Design review of the part built by this model. Coordinates are the model's own, in mm. Face numbers are marked on the shaded views. A direction names the side the tool comes from. Coordinates: 2 decimals unless noted, no trailing zeros. Order: outer loops, then holes, each group sorted by start corner. A loop starts at its lowest first (then second) coordinate and runs counter-clockwise, first axis right, second up.
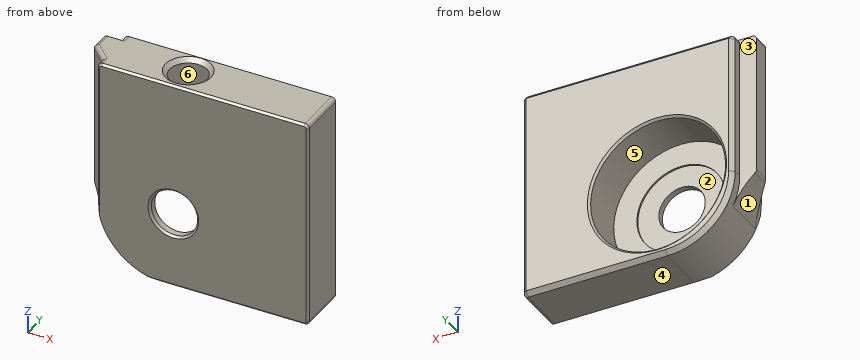
from build123d import *

# Parameters (mm, degrees)
SKETCH1_W           = 25
SKETCH1_H           = 25
BOSS_EXTRUDE1_DEPTH = 6.5
SKETCH2_R           = 8
CUT_EXTRUDE1_DEPTH  = 5.5
FILLET1_R           = 8
SKETCH4_R           = 2.2
CUT_EXTRUDE2_DEPTH  = 7.5
BOSS_EXTRUDE2_DEPTH = 17
FILLET2_R           = 10
SKETCH6_R           = 2.75
CUT_EXTRUDE3_DEPTH  = 20.918584287
BOSS_EXTRUDE3_START = 0.2
SKETCH7_R           = 8
SKETCH7_R_2         = 5.25
BOSS_EXTRUDE3_DEPTH = 0.2
FILLET3_R           = 0.5
CHAMFER1_SIZE       = 0.5
CHAMFER7_SIZE       = 0.25


# Some blends are built 0.0001 mm under size
with BuildPart() as part:
    # Sketch1 → Boss-Extrude1 (new body)
    with BuildSketch(Plane(origin=(0, 0, 0), x_dir=(1, 0, 0), z_dir=(0, 1, 0))):
        Rectangle(SKETCH1_W, SKETCH1_H)
    extrude(amount=BOSS_EXTRUDE1_DEPTH)

    # Sketch2 → Cut-Extrude1 (cut)
    with BuildSketch(Plane(origin=(0, 6.5, 0), x_dir=(1, 0, 0), z_dir=(0, 1, 0))):
        with Locations(Location((-3.5, 3.5, 0), (0, 0, 270))):
            Circle(SKETCH2_R)
    extrude(amount=-CUT_EXTRUDE1_DEPTH, mode=Mode.SUBTRACT)

    # Fillet1
    fillet1_edges = [part.edges().sort_by_distance(p)[0] for p in [
        (-12.5, 3.25, -12.5),
    ]]
    fillet(fillet1_edges, radius=FILLET1_R)

    # Sketch4 → Cut-Extrude2 (cut)
    with BuildSketch(Plane.XY.offset(12.5)):
        with Locations((-3.5, 3.25)):
            Circle(SKETCH4_R)
    extrude(amount=-CUT_EXTRUDE2_DEPTH, mode=Mode.SUBTRACT)

    # Sketch5 → Boss-Extrude2 (add)
    with BuildSketch(Plane.XY.offset(12.5)):
        Polygon((-12.5, 1), (-14.5, 3), (-14.5, 5), (-12.5, 5), align=None)
    extrude(amount=-BOSS_EXTRUDE2_DEPTH)

    # Fillet2
    # the kernel refuses this fillet: 10 mm, written as the material it adds along each edge
    with BuildSketch(Plane(origin=(-12.5, 5, -4.5), x_dir=(0.22360679774997813, 0, -0.9746794344808967), z_dir=(0, -1, 0))) as fillet2_piece_1_section:
        with BuildLine():
            CenterArc((5.813776741, -9.746794345), FILLET2_R, 102.920966382, 25.841932763)
            Line((-0.447213595, -1.949358869), (-0.572433402, -1.793410159))
            ThreePointArc((-0.572433402, -1.793410159), (-0.418542685, -0.929958075), (-0.194935887, 0.04472136))
            Line((-0.194935887, 0.04472136), (0.04472136, 0.194935887))
            ThreePointArc((0.04472136, 0.194935887), (1.788854382, -0.002564524), (3.532987404, 0.194935887))
            Line((3.532987404, 0.194935887), (3.577708764, 0))
        make_face()
    fillet2_piece_1 = extrude(amount=12.94427191, mode=Mode.PRIVATE)
    fillet2_piece_1 = split(fillet2_piece_1, bisect_by=Plane(origin=(-14.5, 3, -4.5), z_dir=(0.7071067811865512, 0.7071067811865438, 0)), keep=Keep.TOP, mode=Mode.PRIVATE)
    add(fillet2_piece_1)

    # Sketch6 → Cut-Extrude3 (cut, through all)
    with BuildSketch(Plane(origin=(0, 1, 0), x_dir=(1, 0, 0), z_dir=(0, 1, 0))):
        with Locations(Location((-3.5, 3.5, 0), (0, 0, 270))):
            Circle(SKETCH6_R)
    extrude(amount=-CUT_EXTRUDE3_DEPTH, mode=Mode.SUBTRACT)

    # Sketch7 → Boss-Extrude3 (add)
    with BuildSketch(Plane(origin=(0, 1, 0), x_dir=(1, 0, 0), z_dir=(0, 1, 0)).offset(BOSS_EXTRUDE3_START)):
        with Locations(Location((-3.5, 3.5, 0), (0, 0, 270))):
            Circle(SKETCH7_R)
        with Locations(Location((-3.5, 3.5, 0), (0, 0, 270))):
            Circle(SKETCH7_R_2, mode=Mode.SUBTRACT)
    extrude(amount=-BOSS_EXTRUDE3_DEPTH)

    # Fillet3
    fillet3_edges = [part.edges().sort_by_distance(p)[0] for p in [
        (-14.5, 4, -4.5),
        (-12.5, 0.5, 12.5),
        (-13.5, 2, 12.5),
        (-14.5, 4, 12.5),
        (-12.5, 5.75, 12.5),
        (12.5, 3.25, -12.5),
        (12.5, 3.25, 12.5),
    ]]
    fillet(fillet3_edges, radius=FILLET3_R)

    # Chamfer1
    chamfer1_edges = [part.edges().sort_by_distance(p)[0] for p in [
        (0, 6.5, 12.5),
        (3.75, 6.5, -12.5),
        (12.5, 6.5, 0),
        (12.353553391, 6.5, 12.353553391),
        (12.353553391, 6.5, -12.353553391),
        (-12.353553391, 6.5, 12.353553391),
        (-12.5, 6.5, 3.75),
        (-10.156854249, 6.5, -10.156854249),
        (-5.7, 3.25, 12.5),
    ]]
    chamfer(chamfer1_edges, length=CHAMFER1_SIZE - 0.0001)  # a hair under: the kernel refuses the full size

    # Chamfer7
    # the kernel refuses this chamfer: 0.25 mm, written as the material it takes off along each edge
    with BuildSketch(Plane(origin=(-3.5, 0, -3.5), x_dir=(0, 0, 1), z_dir=(-1, 0, 0))) as chamfer7_piece_1:
        Polygon((2.75 + CHAMFER7_SIZE, 0), (2.75, CHAMFER7_SIZE), (2.75, 0), align=None)
    revolve(axis=Axis((-3.5, 0, -3.5), (0, 1, 0)), mode=Mode.SUBTRACT)
    with BuildSketch(Plane(origin=(-12.5, 0, -7.714603735), x_dir=(1, 0, 0), z_dir=(0, 0, 1)), Plane(origin=(12, 0, -12.5), x_dir=(0, 0, 1), z_dir=(-1, 0, 0))) as chamfer7_piece_2:
        Polygon((CHAMFER7_SIZE, 0), (0, CHAMFER7_SIZE), (0, 0), align=None)
    extrude(amount=19.714603735, mode=Mode.SUBTRACT)
    with BuildSketch(Plane(origin=(-12, 0, 12.5), x_dir=(0, 1, 0), z_dir=(1, 0, 0))) as chamfer7_piece_3:
        Polygon((CHAMFER7_SIZE, 0), (0, -CHAMFER7_SIZE), (0, 0), align=None)
    extrude(amount=24, mode=Mode.SUBTRACT)
    with BuildSketch(Plane(origin=(12.5, 0, 12), x_dir=(-1, 0, 0), z_dir=(0, 0, -1))) as chamfer7_piece_4:
        Polygon((CHAMFER7_SIZE, 0), (0, CHAMFER7_SIZE), (0, 0), align=None)
    extrude(amount=24, mode=Mode.SUBTRACT)
    with BuildSketch(Plane(origin=(-3.5, 6.5, -3.5), x_dir=(0, 0, 1), z_dir=(-1, 0, 0))) as chamfer7_piece_5:
        Polygon((8 + CHAMFER7_SIZE, 0), (8, -CHAMFER7_SIZE), (8, 0), align=None)
    revolve(axis=Axis((-3.5, 6.5, -3.5), (0, 1, 0)), mode=Mode.SUBTRACT)
    with BuildSketch(Plane(origin=(12, 0, -12), x_dir=(0, 0, -1), z_dir=(-1, 0, 0))) as chamfer7_piece_6:
        Polygon((0.5 - CHAMFER7_SIZE, 0), (0.5, -CHAMFER7_SIZE), (0.5, 0), align=None)
    revolve(axis=Axis((12, 0, -12), (0, -1, 0)), revolution_arc=90, mode=Mode.SUBTRACT)
    with BuildSketch(Plane(origin=(12, 0, 12), x_dir=(0, 0, 1), z_dir=(-1, 0, 0))) as chamfer7_piece_7:
        Polygon((0.5, CHAMFER7_SIZE), (0.5 - CHAMFER7_SIZE, 0), (0.5, 0), align=None)
    revolve(axis=Axis((12, 0, 12), (0, 1, 0)), revolution_arc=90, mode=Mode.SUBTRACT)
    with BuildSketch(Plane(origin=(-12, 0, 12), x_dir=(0, 0, 1), z_dir=(1, 0, 0))) as chamfer7_piece_8:
        Polygon((0.5 - CHAMFER7_SIZE, 0), (0.5, -CHAMFER7_SIZE), (0.5, 0), align=None)
    revolve(axis=Axis((-12, 0, 12), (0, -1, 0)), revolution_arc=90, mode=Mode.SUBTRACT)


solid = part.part
1. Add section A-A (z = -3.5). Give the boundary of the cut face in (x, y), and give its area (3 significant figures).
2. To check wall thickness, follow line 1 (X direction, y = 0.85, z = -3.5); line 2 (Y direction, x = -3.5, z = 10); line 3 (Y direction, x = -1.75, z = 1.5). State the ranges of each line that lie inside material, in increasing order.
3. Add section C-C (z = 10.75). Give the boundary of the cut face in (x, y), and give its area (3 significant figures).
4. For the marked faces 4, 5 and 6, list the 3-axis set-ups (+Z, -Z, +X, -X, +Y, -Y) from which the entire face can be reached by the end or side of a thin tool; tool diameter is ignored.
5. Mouldability with a two-part tool opening along Z and no side actions: class the marked faces 1, 2 and 3 as pulls with the +Z half, pulls with the -Z half, needs draft (parallel to the pull), parting line crosses it, or undercut.
6. Insertion check: pin 1 (0.8 mm diameter, centred on y = 5.5, z = 3.5, fed in from -X); pin 2 (2 mm diameter, centred on x = -6, z = 2, fed in from -Y); pin 3 (3.5 mm diameter, centred on x = -3.5, z = -3.5, fed in from +Y); pin 4 (0.8 mm diameter, centred on x = -13.5, z = 5.5, fed in from +Y). Each pin has a flat end and moves straight along its axis. Give the tip position at first contact, or say it passes through.
Solution:
1. outline: (-14.5, 3) - (-12.5, 1) - (-12.5, 0.25) - (-12.25, 0) - (-6.5, 0) - (-6.25, 0.25) - (-6.25, 1) - (-8.75, 1) - (-8.75, 1.2) - (-11.5, 1.2) - (-11.5, 6.25) - (-11.75, 6.5) - (-12, 6.5) - (-12.5, 6) - (-12.5, 5) - (-14.5, 5) - close; (-0.75, 0.25) - (-0.5, 0) - (12.25, 0) - (12.5, 0.25) - (12.5, 6) - (12, 6.5) - (4.75, 6.5) - (4.5, 6.25) - (4.5, 1.2) - (1.75, 1.2) - (1.75, 1) - (-0.75, 1) - close
1. area: 75.7 mm2
2. line 1: x = -12.5 to -6.25, -0.75 to 12.5
2. line 2: y = 0 to 1.05, 5.45 to 6.5
2. line 3: y = 0 to 1.2
3. outline: (-14.5, 3) - (-12.5, 1) - (-12.5, 0.25) - (-12.25, 0) - (12.25, 0) - (12.5, 0.25) - (12.5, 6) - (12, 6.5) - (-12, 6.5) - (-12.5, 6) - (-12.5, 5) - (-14.5, 5) - close; hole circle Ø4.4 at (-3.5, 3.25)
3. area: 153 mm2
4. face 4: -Z, +X, -X, +Y, -Y
4. face 5: +Y
4. face 6: +Z
5. face 1: pulls with the -Z half
5. face 2: undercut
5. face 3: needs draft
6. pin 1: stops at x = -12.5
6. pin 2: stops at y = 0
6. pin 3: passes through
6. pin 4: stops at y = 5
